Here's how the part is built. I have some questions about the finished solid (model axes, mm). Round coordinates to 2 decimals unless told otherwise and drop trailing zeros. Write each loop counter-clockwise with the first axis right and the second up, starting at its lowest first coordinate (ties: lowest second). Pieces come first, ordered by that corner, then holes. Notation, with made-up numbers: M 34,67.25 L 65,67.25 A13 ccw 65,83.25 Z; hole C 62,84.5 d1. An arc over 180 degrees is marked long. Use one line per item in the form item = value. Start each with the question number.
Q1. We'd pull the mould along Y, two halves only. Please class faces 1 (the face through (2.02, 2.345, 0.738)), 2 (the face through (1.972, -4.35, -2.465)), 3 (the face through (1.972, 4.31, -2.535)): +Y half, -Y half, draft (parallel to the pull), parting line (faces both ways), or undercut.
Q2. I want a section at B-B on x = 3.7. List the corners of the cut face in (y, z) for me.
Q3. I need wall thicknesses on line 1 along Z through (x, y) = (1.9, 0); line 2 along Y through (x, z) = (3.15, 1.5); line 3 along Z through (x, y) = (0.95, 2.25). Which ranges of each line are inside material? Lowest first, please. Write a range as from..to.
Q4. I want a section at A-A on x = 1.9. List the corners of the cut face in (y, z) for me.
Autodesk Inventor part; units mm, degrees
ref_plane "DADO1_XY" through (0, 0, 0) normal (1, 0, 0) x (0, 0, -1)
ref_plane "DADO1_YZ" through (0, 0, 0) normal (0, 0, -1) x (0, 1, 0)
ref_plane "DADO1_ZX" through (0, 0, 0) normal (0, 1, 0) x (1, 0, 0)
sketch "Skizze_1" plane through (0, 0, 0) normal (0, 0, 1) x (1, 0, 0)
  line L0 (4, 0) -> (0, 0)
  line L1 (0, 0) -> (0, 5)
  line L2 (0, 5) -> (0.5774, 6)
  line L3 (0.5774, 6) -> (3.4226, 6)
  line L4 (3.4226, 6) -> (4, 5)
  line L5 (4, 5) -> (4, 0)
  line L6 (4, 0) -> (0, 0)
revolve "Revolution1" add sketch "Skizze_1" angle 360 about axis through (4, 0, 0) along (1, 0, 0)
sketch "Skizze_2_ALT_Drilling_1" plane through (0, 0, 0) normal (0, 0, 1) x (1, 0, 0)
  line L0 (4, 0) -> (0, 0)
  line L1 (0, 0) -> (0, 3)
  line L2 (0, 3) -> (0.5415, 2.4585)
  line L3 (0.5415, 2.4585) -> (3.4585, 2.4585)
  line L4 (3.4585, 2.4585) -> (4, 3)
  line L5 (4, 3) -> (4, 0)
  line L6 (4, 0) -> (0, 0)
revolve "Revolution2" cut sketch "Skizze_2_ALT_Drilling_1" angle 360 about axis through (4, 0, 0) along (1, 0, 0)
thread "Thread1"
sketch "Skizze_3" plane through (0, 0, 0) normal (1, 0, 0) x (0, 1, 0)
  line L0 (-10, 10) -> (-10, -10)
  line L1 (-10, -10) -> (10, -10)
  line L2 (10, -10) -> (10, 10)
  line L3 (10, 10) -> (-10, 10)
  line L4 (-2.8868, 5) -> (-5.7735, 0)
  line L5 (-5.7735, 0) -> (-2.8868, -5)
  line L6 (-2.8868, -5) -> (2.8868, -5)
  line L7 (2.8868, -5) -> (5.7735, 0)
  line L8 (5.7735, 0) -> (2.8868, 5)
  line L9 (2.8868, 5) -> (-2.8868, 5)
extrude "Extrusion1" cut sketch "Skizze_3" along normal blind 4
ref_plane "DADO1_XY" through (0, 0, 0) normal (1, 0, 0) x (0, 0, -1)
ref_plane "DADO1_YZ" through (0, 0, 0) normal (0, 0, -1) x (0, 1, 0)
ref_plane "DADO1_ZX" through (0, 0, 0) normal (0, 1, 0) x (1, 0, 0)
properties part number "U-12-16"
Reported:
q1.face_1 = undercut
q1.face_2 = -Y half
q1.face_3 = +Y half
q2.outline = M -5.5,-0.48 L -3.16,-4.52 A5.52 ccw -2.34,-5 L 2.34,-5 A5.52 ccw 3.16,-4.52 L 5.5,-0.48 A5.52 ccw 5.5,0.48 L 3.16,4.52 A5.52 ccw 2.34,5 L -2.34,5 A5.52 ccw -3.16,4.52 L -5.5,0.48 A5.52 ccw Z; hole C 0,0 d5.4
q3.line_1 = -5..-2.46, 2.46..5
q3.line_2 = -4.91..-1.95, 1.95..4.91
q3.line_3 = -5..-0.99, 0.99..5
q4.outline = M -5.77,0 L -2.89,-5 L 2.89,-5 L 5.77,0 L 2.89,5 L -2.89,5 Z; hole C 0,0 d4.92
